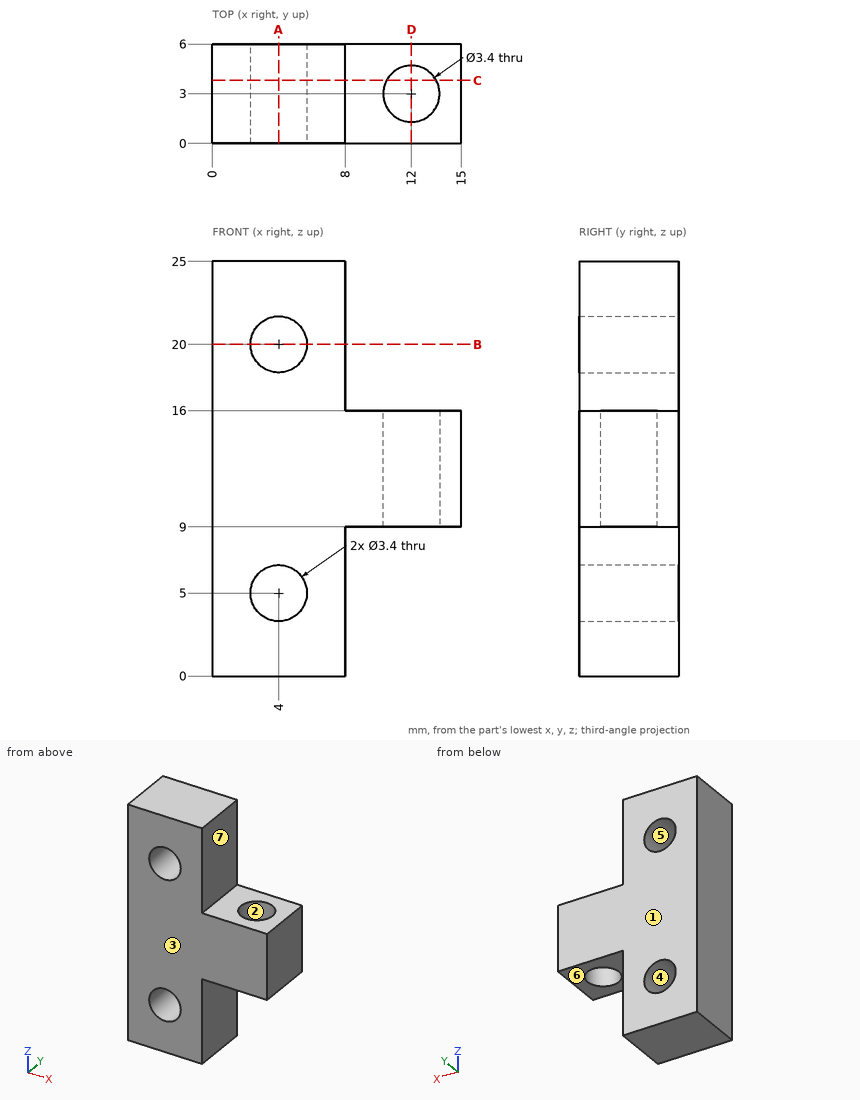
Answer from the drawing. Dimensions are ordinates in mm from the lowest x, y and z of the part. A direction names the side the tool comes from. Give positions to 0.01 mm unless a question says otherwise; leave off trailing zeros. Loops run counter-clockwise (first coordinate to the right, second up) from the corner with the lowest first, then second, coordinate; pieces in that order, holes last. Notation, with made-up numbers: (59.5, 19) -> (69.5, 19) arc R33 ccw to (69.5, 56) -> close; hole circle Ø1 at (37, 17.5). An arc over 180 degrees is marked (long way). One line per question, with ' | ' between items. Start each with the question number.
1) Straight lines are drawn through the part: L1, parallel to Z at x = 4, y = 2.65; L2, parallel to X at y = 3.7, z = 20; L3, parallel to Y at x = 12, z = 11.75. For each, find the intervals that lie inside material, in ascending order.
2) Each of these flat-tipped pins is pushed along its axis until it touches: pin 1 (3 mm diameter, centred on x = 4, z = 5, fed in from +Y); pin 2 (3 mm diameter, centred on x = 12.5, y = 2.5, fed in from -Z). Where does it stop, or does it pass through?
3) Section A-A, the plane x = 4 is taken. Determine the outline of the cut face in (y, z).
4) Section D-D, the plane x = 12 is taken. Determine the outline of the cut face in (y, z).
5) For the marked faces 5, 6 and 7, determine the directions among +Z, -Z, +X, -X, +Y, -Y from which every point of the face is accessible in a straight line to the end or side of a thin tool.
6) Section B-B, the plane z = 20 is taken. Determine the outline of the cut face in (x, y), then the cut area to 3 significant figures.
7) Section C-C, the plane y = 3.8 is taken. Determine the outline of the cut face in (x, z).
8) Determine the mould class of the marked faces 1, 2, 3 and 4 for opening direction Y: +Y half, -Y half, draft (parallel to the pull), parting line (faces both ways), or undercut.
Resolved:
1) L1: 0 to 3.3, 6.7 to 18.3, 21.7 to 25 | L2: 0 to 2.3, 5.7 to 8 | L3: 0 to 1.3, 4.7 to 6
2) pin 1: through | pin 2: z = 9
3) outline: (0, 0) -> (6, 0) -> (6, 3.3) -> (0, 3.3) -> close; (0, 6.7) -> (6, 6.7) -> (6, 18.3) -> (0, 18.3) -> close; (0, 21.7) -> (6, 21.7) -> (6, 25) -> (0, 25) -> close
4) outline: (0, 9) -> (1.3, 9) -> (1.3, 16) -> (0, 16) -> close; (4.7, 9) -> (6, 9) -> (6, 16) -> (4.7, 16) -> close
5) face 5: +Y, -Y | face 6: -Z, +X, +Y, -Y | face 7: +Z, +X, +Y, -Y
6) outline: (0, 0) -> (2.3, 0) -> (2.3, 6) -> (0, 6) -> close; (5.7, 0) -> (8, 0) -> (8, 6) -> (5.7, 6) -> close | area: 27.6 mm2
7) outline: (0, 0) -> (8, 0) -> (8, 9) -> (10.5, 9) -> (10.5, 16) -> (8, 16) -> (8, 25) -> (0, 25) -> close; (13.5, 9) -> (15, 9) -> (15, 16) -> (13.5, 16) -> close; hole circle Ø3.4 at (4, 5); hole circle Ø3.4 at (4, 20)
8) face 1: +Y half | face 2: undercut | face 3: -Y half | face 4: draft
